```python
from build123d import *

# Parameters (mm, degrees)
FILLET1_R = 2
FILLET2_R = 2


with BuildPart() as part:
    # Sketch1 → Revolve1 (revolve)
    with BuildSketch(Plane.XY):
        Polygon((0, 0), (3, 0), (3, 5), (2, 9), (0, 9), align=None)
    revolve(axis=Axis((0, 9, 0), (0, -1, 0)))

    # Fillet1
    fillet1_edges = [part.edges().sort_by_distance(p)[0] for p in [
        (-2, 9, 0),
    ]]
    fillet(fillet1_edges, radius=FILLET1_R)

    # Fillet2
    fillet2_edges = [part.edges().sort_by_distance(p)[0] for p in [
        (-3, 5, 0),
    ]]
    fillet(fillet2_edges, radius=FILLET2_R)


solid = part.part
```
Geometry: final body of the model. Coordinates: model frame, mm. Coordinates: 2 decimals unless noted, no trailing zeros. Order: outer loops, then holes, each group sorted by start corner. A loop starts at its lowest first (then second) coordinate and runs counter-clockwise, first axis right, second up. Notation, with made-up numbers: (75.5, 32) -> (110.5, 32) arc R21 cw to (110.5, 51) -> close; hole circle Ø4 at (75, -7.5). An arc over 180 degrees is marked (long way). Write each question's results on one line, items separated by ' | '. Start each with the question number.
1) First-contact query: pin 1 (1.5 mm diameter, centred on y = 7, z = -1.5, fed in from -X); pin 2 (2 mm diameter, centred on x = -1.5, y = 4.5, fed in from -Z). Flat tips, straight axial feed; report the tip coordinate or a pass-through.
2) Cut plane A-A, the plane y = 6. Output: boundary loops of the cut face in (x, z), and give its area (3 significant figures).
3) Cut plane B-B, the plane y = 1.25. Output: boundary loops of the cut face in (x, z).
4) Material intervals for line 1 along X through (y, z) = (7, 0); line 2 along Y through (x, z) = (-1, 0.5); line 3 along Z through (x, y) = (-2, 2), sorted ascending.
Checks:
1) pin 1: x = -2.45 | pin 2: z = -2.96
2) outline: circle Ø5.5 at (0, 0) | area: 23.8 mm^2
3) outline: circle Ø6 at (0, 0)
4) line 1: -2.5 to 2.5 | line 2: 0 to 8.88 | line 3: -2.24 to 2.24
